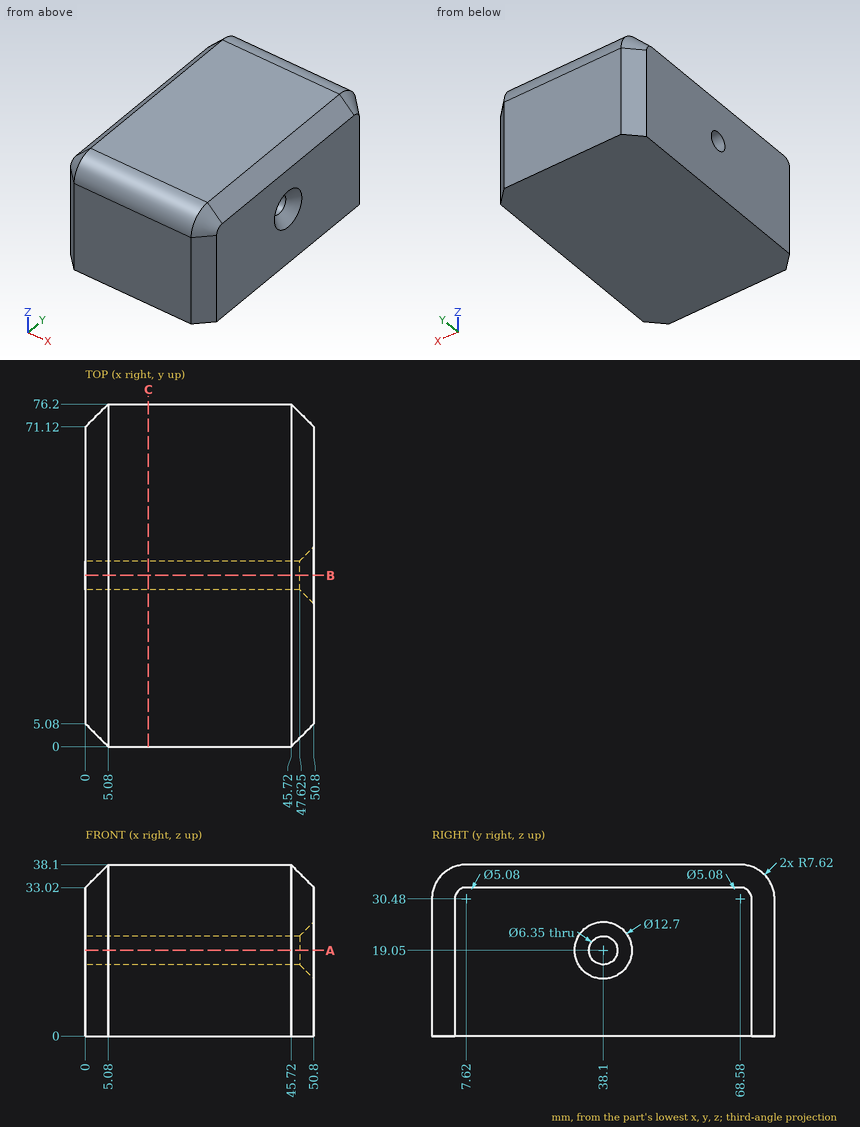
Answer from the drawing. Dimensions are ordinates in mm from the lowest x, y and z of the part. Coordinates: 2 decimals unless noted, no trailing zeros. Loops run counter-clockwise (first coordinate to the right, second up) from the corner with the lowest first, then second, coordinate; pieces in that order, holes last. Notation, with made-up numbers: (15.25, 41.5) -> (46.25, 41.5) arc R20 cw to (46.25, 64.5) -> close; hole circle Ø6 at (17, -38). An arc over 180 degrees is marked (long way). Answer in a Markdown table with one row per item.
Item 1: A cutting plane is placed at A-A on z = 19.05. Determine the outline of the cut face in (x, y) (3 decimals).
Returned:
| item | result |
|---|---|
| outline | (0, 5.08) -> (5.08, 0) -> (45.72, 0) -> (50.8, 5.08) -> (50.8, 31.75) -> (47.625, 34.925) -> (0, 34.925) -> close; (0, 41.275) -> (47.625, 41.275) -> (50.8, 44.45) -> (50.8, 71.12) -> (45.72, 76.2) -> (5.08, 76.2) -> (0, 71.12) -> close |
Item 2: A cutting plane is placed at C-C on x = 14. Determine the outline of the cut face in (y, z) (3 decimals).
Returned:
| item | result |
|---|---|
| outline | (0, 0) -> (76.2, 0) -> (76.2, 30.48) arc R7.62 ccw to (68.58, 38.1) -> (7.62, 38.1) arc R7.62 ccw to (0, 30.48) -> close; hole circle Ø6.35 at (38.1, 19.05) |
Item 3: Straight lines are drawn through the part: line 1 along Z through (x, y) = (31, 38); line 2 along Z through (x, y) = (10.5, 36); line 3 along Z through (x, y) = (14, 7.5). For each, find the intervals that lie inside material, in ascending order. Write a range as [from, to].
Returned:
| item | result |
|---|---|
| line 1 | z = [0, 15.88], [22.22, 38.1] |
| line 2 | z = [0, 16.67], [21.43, 38.1] |
| line 3 | z = [0, 38.1] |
Item 4: A cutting plane is placed at B-B on y = 38.1. Determine the outline of the cut face in (x, z) (3 decimals).
Returned:
| item | result |
|---|---|
| outline | (0, 0) -> (50.8, 0) -> (50.8, 12.7) -> (47.625, 15.875) -> (0, 15.875) -> close; (0, 22.225) -> (47.625, 22.225) -> (50.8, 25.4) -> (50.8, 33.02) -> (45.72, 38.1) -> (5.08, 38.1) -> (0, 33.02) -> close |
